Geometry check sheet. Reference: the model listing, model coordinates, mm. A direction names the side the tool comes from. Coordinates: 2 decimals unless noted, no trailing zeros. Write each loop counter-clockwise with the first axis right and the second up, starting at its lowest first coordinate (ties: lowest second). Pieces come first, ordered by that corner, then holes. Notation, with made-up numbers: M -10,20 L 35,20 A6 cw 35,24 Z; hole C -8.75,-19.75 d10. An arc over 180 degrees is marked long. Put each result on its own line as item: value. Start each with the question number.
1) Cross-section at D-D on y = -20. Record the cut outline in (x, z).
2) Scan lines: line 1 along X through (y, z) = (17.5, 6.25); line 2 along Y through (x, z) = (0, 5); line 3 along X through (y, z) = (17, 2). Record each from-to range of solid material in increasing order.
3) Mould release check, pull along Y, two halves, no side actions. Record for faces 1 (the cylindrical face through (-34.514, 18.053, 4.93)), 2 (the cylindrical face through (-16.8, 36.3, 4.9)), 3 (the flat face through (30, 18, 10)), 4 (the flat face through (28.31, -26.966, 4.93)): released by +Y, released by -Y, zero draft, split by the parting line, or undercut.
4) Cross-section at A-A on y = 20. Record the cut outline in (x, z), plus the area to 3 significant figures.
5) Cross-section at C-C on z = 21.5. Record the cut outline in (x, y), plus the area to 3 significant figures.
6) Set-up check for faces 5 (the flat face through (0, 36, 10)), 6 (the flat face through (1, -40, 48)), 7 (the flat face through (-37.51, -11.03, 4.93)), 8 (the cylindrical face through (34.45, 18.42, 4.93)), 9 (the cylindrical face through (-38.373, 11.291, 4.93)): record each of +Z, -Z, +X, -X, +Y, -Y from which the full face is reachable in a straight line by a thin tool's end or side.
7) Cross-section at B-B on x = 24.5. Record the cut outline in (y, z), plus the area to 3 significant figures.
8) Gauge pin test, flat ends, axial feed: pin 1 (13.5 mm diameter, centred on x = 30.3, y = 17.5, fed in from -Z); pin 2 (7.5 mm diameter, centred on x = 0, y = -35, fed in from +Z); pin 3 (5 mm diameter, centred on x = -30.3, y = 17.5, fed in from -Z); pin 4 (10 mm diameter, centred on x = 17, z = 41, fed in from +Y). Record the tip position at first contact, or that the pin passes through.
from build123d import *

# Parameters (mm, degrees)
ESTRUSIONE_ESTRUSIONE2_DEPTH = 10
ESTRUSIONE_ESTRUSIONE3_DEPTH = 50


with BuildPart() as part:
    # Schizzo4 → Estrusione-Estrusione2 (new body)
    with BuildSketch(Plane.XY):
        with BuildLine():
            ThreePointArc((5.811411188, 38), (0, 34.05), (-5.811411188, 38))
            Line((-5.811411188, 38), (-12.489995997, 38))
            ThreePointArc((-12.489995997, 38), (-16.909196271, 36.250228709), (-21.089648938, 33.988626151))
            Line((-21.089648938, 33.988626151), (-17.322367371, 29.336420856))
            ThreePointArc((-17.322367371, 29.336420856), (-16.844140316, 27.721953377), (-17.647583626, 26.242194881))
            Line((-17.647583626, 26.242194881), (-21.99960101, 22.718000691))
            ThreePointArc((-21.99960101, 22.718000691), (-23.61406849, 22.239773636), (-25.093826986, 23.043216946))
            Line((-25.093826986, 23.043216946), (-28.861108553, 27.695422241))
            ThreePointArc((-28.861108553, 27.695422241), (-38.449109313, 11.03023087), (-39.153963342, -8.183346174))
            Line((-39.153963342, -8.183346174), (-35.814606143, -13.967282507))
            ThreePointArc((-35.814606143, -13.967282507), (-29.487341226, -17.025), (-30.002912658, -24.033430901))
            Line((-30.002912658, -24.033430901), (-26.663967345, -29.816653826))
            ThreePointArc((-26.663967345, -29.816653826), (0, -40), (26.663967345, -29.816653826))
            Line((26.663967345, -29.816653826), (30.002912658, -24.033430901))
            ThreePointArc((30.002912658, -24.033430901), (29.487341226, -17.025), (35.814606143, -13.967282507))
            Line((35.814606143, -13.967282507), (39.153963342, -8.183346174))
            ThreePointArc((39.153963342, -8.183346174), (34.641016151, 20), (12.489995997, 38))
            Line((12.489995997, 38), (5.811411188, 38))
        make_face()
        with BuildLine():
            ThreePointArc((-9, -33.621), (-10.621, -32), (-9, -30.379))
            ThreePointArc((-9, -30.379), (-7.379, -32), (-9, -33.621))
        make_face(mode=Mode.SUBTRACT)
        with BuildLine():
            ThreePointArc((9, -33.621), (7.379, -32), (9, -30.379))
            ThreePointArc((9, -30.379), (10.621, -32), (9, -33.621))
        make_face(mode=Mode.SUBTRACT)
        with BuildLine():
            ThreePointArc((-30.3, 21.75), (-26.05, 17.5), (-30.3, 13.25))
            ThreePointArc((-30.3, 13.25), (-34.55, 17.5), (-30.3, 21.75))
        make_face(mode=Mode.SUBTRACT)
        with BuildLine():
            ThreePointArc((30.3, 21.75), (34.55, 17.5), (30.3, 13.25))
            ThreePointArc((30.3, 13.25), (26.05, 17.5), (30.3, 21.75))
        make_face(mode=Mode.SUBTRACT)
        with BuildLine():
            ThreePointArc((0, -30.75), (4.25, -35), (0, -39.25))
            ThreePointArc((0, -39.25), (-4.25, -35), (0, -30.75))
        make_face(mode=Mode.SUBTRACT)
        with BuildLine():
            ThreePointArc((-35, -3.5), (-38.5, 0), (-35, 3.5))
            ThreePointArc((-35, 3.5), (-31.5, 0), (-35, -3.5))
        make_face(mode=Mode.SUBTRACT)
        with BuildLine():
            ThreePointArc((35, -3.5), (31.5, 0), (35, 3.5))
            ThreePointArc((35, 3.5), (38.5, 0), (35, -3.5))
        make_face(mode=Mode.SUBTRACT)
        with BuildLine():
            ThreePointArc((0, 27.5), (27.5, 0), (0, -27.5))
            ThreePointArc((0, -27.5), (-27.5, 0), (0, 27.5))
        make_face(mode=Mode.SUBTRACT)
        with BuildLine():
            ThreePointArc((25, 22.933), (22.933, 25), (25, 27.067))
            ThreePointArc((25, 27.067), (27.067, 25), (25, 22.933))
        make_face(mode=Mode.SUBTRACT)
        with BuildLine():
            ThreePointArc((0, -27.5), (-27.5, 0), (0, 27.5))
            ThreePointArc((0, 27.5), (27.5, 0), (0, -27.5))
        make_face()
        with BuildLine():
            ThreePointArc((-35, 3.5), (-31.5, 0), (-35, -3.5))
            ThreePointArc((-35, -3.5), (-38.5, 0), (-35, 3.5))
        make_face()
        with BuildLine():
            ThreePointArc((9, -30.379), (10.621, -32), (9, -33.621))
            ThreePointArc((9, -33.621), (7.379, -32), (9, -30.379))
        make_face()
        with BuildLine():
            ThreePointArc((-9, -30.379), (-7.379, -32), (-9, -33.621))
            ThreePointArc((-9, -33.621), (-10.621, -32), (-9, -30.379))
        make_face()
        with BuildLine():
            ThreePointArc((35, 3.5), (38.5, 0), (35, -3.5))
            ThreePointArc((35, -3.5), (31.5, 0), (35, 3.5))
        make_face()
        with BuildLine():
            ThreePointArc((25, 27.067), (27.067, 25), (25, 22.933))
            ThreePointArc((25, 22.933), (22.933, 25), (25, 27.067))
        make_face()
    extrude(amount=ESTRUSIONE_ESTRUSIONE2_DEPTH)

    # Schizzo5 → Estrusione-Estrusione3 (add, symmetric)
    with BuildSketch(Plane(origin=(0, 0, 0), x_dir=(0, 0, -1), z_dir=(1, 0, 0))):
        Polygon((-10, 38), (-10, -40), (-88, -40), align=None)
    extrude(amount=ESTRUSIONE_ESTRUSIONE3_DEPTH, both=True)


solid = part.part
Answer key:
1. outline: M -50,10 L -28.65,10 L -28.65,0 L 28.65,0 L 28.65,10 L 50,10 L 50,68 L -50,68 Z
2. line 1: x = -35.97 to -34.55, -26.05 to 26.05, 34.55 to 35.97
2. line 2: y = -40 to -39.25, -30.75 to 34.05
2. line 3: x = -36.21 to -34.52, -26.08 to 26.08, 34.52 to 36.21
3. face 1: undercut
3. face 2: released by +Y
3. face 3: undercut
3. face 4: released by -Y
4. outline: M -50,10 L -34.64,10 L -34.64,0 L -33.74,0 L -33.74,10 L -26.86,10 L -26.86,0 L 26.86,0 L 26.86,10 L 33.74,10 L 33.74,0 L 34.64,0 L 34.64,10 L 50,10 L 50,28 L -50,28 Z
4. area: 2,360 mm²
5. outline: M -50,-40 L 50,-40 L 50,26.5 L -50,26.5 Z
5. area: 6,650 mm²
6. face 5: -Z, +Y
6. face 6: +Z, -Z, +X, -X, -Y
6. face 7: -Z, -X, -Y
6. face 8: -Z
6. face 9: -Z, -X
7. outline: M -40,10 L -31.62,10 L -31.62,0 L 31.62,0 L 31.62,10 L 38,10 L -40,88 Z
7. area: 3,670 mm²
8. pin 1: stops at z = 0
8. pin 2: stops at z = 86.75
8. pin 3: stops at z = 10
8. pin 4: stops at y = 12
